```python
from build123d import *

# Parameters (mm, degrees)
SKETCH_1_R      = 38
SKETCH_1_R_2    = 5
SKETCH_1_R_3    = 2.5
SKETCH_1_R_4    = 1.5
EXTRUDE_2_DEPTH = 4


with BuildPart() as part:
    # 草图1 → 凸台-拉伸2 (new body)
    with BuildSketch(Plane.XY):
        Circle(SKETCH_1_R)
        Circle(SKETCH_1_R_2, mode=Mode.SUBTRACT)
        with Locations((0, 30)):
            Circle(SKETCH_1_R_3, mode=Mode.SUBTRACT)
        with Locations((21.213203436, 21.213203436)):
            Circle(SKETCH_1_R_3, mode=Mode.SUBTRACT)
        with Locations((30, 0)):
            Circle(SKETCH_1_R_3, mode=Mode.SUBTRACT)
        with Locations((21.213203436, -21.213203436)):
            Circle(SKETCH_1_R_3, mode=Mode.SUBTRACT)
        with Locations((0, -30)):
            Circle(SKETCH_1_R_3, mode=Mode.SUBTRACT)
        with Locations((-21.213203436, -21.213203436)):
            Circle(SKETCH_1_R_3, mode=Mode.SUBTRACT)
        with Locations((-30, 0)):
            Circle(SKETCH_1_R_3, mode=Mode.SUBTRACT)
        with Locations((-21.213203436, 21.213203436)):
            Circle(SKETCH_1_R_3, mode=Mode.SUBTRACT)
        with Locations((0, 14)):
            Circle(SKETCH_1_R_4, mode=Mode.SUBTRACT)
        with Locations((14, 0)):
            Circle(SKETCH_1_R_4, mode=Mode.SUBTRACT)
        with Locations((0, -14)):
            Circle(SKETCH_1_R_4, mode=Mode.SUBTRACT)
        with Locations((-14, 0)):
            Circle(SKETCH_1_R_4, mode=Mode.SUBTRACT)
    extrude(amount=EXTRUDE_2_DEPTH)


solid = part.part
```
Part model, mm, in its own coordinate system. Round coordinates to 2 decimals unless told otherwise and drop trailing zeros. Loops run counter-clockwise (first coordinate to the right, second up) from the corner with the lowest first, then second, coordinate; pieces in that order, holes last.
Item 1: Drop flat-ended pins along their axis: P1, Ø1, axis at y = -28.5, z = 2.5, coming from the -X side; P2, Ø1, axis at y = 17, z = 2.5, coming from the -X side. Give the stop position or say it passes through.
Item 2: Cut at C-C, the plane y = -14. Give the cut face in (x, z), then the cut area to 3 significant figures.
Item 3: Mould opens along Y. For faces 1 (the face through (17.535, -33.713, 1.972)), 2 (the face through (-1, -8, 4)), 3 (the face through (22.56, 23.32, 1.97)) say: +Y half, -Y half, draft (parallel to the pull), parting line (faces both ways), or undercut.
Item 4: Cut at A-A, the plane y = 0. Give the cut face in (x, z), then the cut area to 3 significant figures.
Item 5: Drill centre lines: line 1 (Y direction, x = 0, z = 1.3); line 2 (Y direction, x = -4, z = 0.8); line 3 (X direction, y = 28.5, z = 1). Where is each one in solid material? Low to high.
Item 6: Cut at D-D, the plane x = -29. Give the cut face in (y, z), then the cut area to 3 significant figures.
A:
1. P1: stops at x = -25.69
1. P2: stops at x = -34.23
2. outline: (-35.33, 0) - (-1.5, 0) - (-1.5, 4) - (-35.33, 4) - close; (1.5, 0) - (35.33, 0) - (35.33, 4) - (1.5, 4) - close
2. area: 271 mm2
3. face 1: parting line
3. face 2: draft
3. face 3: undercut
4. outline: (-38, 0) - (-32.5, 0) - (-32.5, 4) - (-38, 4) - close; (-27.5, 0) - (-15.5, 0) - (-15.5, 4) - (-27.5, 4) - close; (-12.5, 0) - (-5, 0) - (-5, 4) - (-12.5, 4) - close; (5, 0) - (12.5, 0) - (12.5, 4) - (5, 4) - close; (15.5, 0) - (27.5, 0) - (27.5, 4) - (15.5, 4) - close; (32.5, 0) - (38, 0) - (38, 4) - (32.5, 4) - close
4. area: 200 mm2
5. line 1: y = -38 to -32.5, -27.5 to -15.5, -12.5 to -5, 5 to 12.5, 15.5 to 27.5, 32.5 to 38
5. line 2: y = -37.79 to -3, 3 to 37.79
5. line 3: x = -25.13 to -2, 2 to 25.13
6. outline: (-24.56, 0) - (-2.29, 0) - (-2.29, 4) - (-24.56, 4) - close; (2.29, 0) - (24.56, 0) - (24.56, 4) - (2.29, 4) - close
6. area: 178 mm2
